from build123d import *

# Parameters (mm, degrees)
BOSS_EXTRUDE1_DEPTH = 1.5875
CUT_EXTRUDE1_DEPTH  = 3.175
FILLET1_R           = 8.89


with BuildPart() as part:
    # Sketch1 → Boss-Extrude1 (new, symmetric)
    with BuildSketch(Plane.XY):
        with BuildLine():
            Line((-120.187952283, -34.272453), (-93.24718392, -61.213221363))
            Line((-93.24718392, -61.213221363), (-94.292689271, -70.797689271))
            ThreePointArc((-94.292689271, -70.797689271), (-77.124658044, -85.289234251), (-57.767453, -96.692952283))
            ThreePointArc((-57.767453, -96.692952283), (94.292689271, 117.787689271), (-120.187952283, -34.272453))
        make_face()
    extrude(amount=BOSS_EXTRUDE1_DEPTH, both=True)

    # Sketch2 → Cut-Extrude1 (cut)
    with BuildSketch(Plane.XY.offset(1.5875)):
        with BuildLine():
            Line((-77.304798152, -55.60299244), (-78.320318415, -64.912577861))
            ThreePointArc((-78.320318415, -64.912577861), (94.997930523, 93.675946819), (-107.51910025, -25.388690342))
            Line((-107.51910025, -25.388690342), (-77.304798152, -55.60299244))
        make_face()
    extrude(amount=-CUT_EXTRUDE1_DEPTH, mode=Mode.SUBTRACT)

    # Fillet1
    fillet1_edges = [part.edges().sort_by_distance(p)[0] for p in [
        (-77.304798152, -55.60299244, 0),
        (-107.51910025, -25.388690342, 0),
        (-78.320318415, -64.912577861, 0),
        (-93.24718392, -61.213221363, -0.79375),
        (-120.187952283, -34.272453, -0.79375),
        (-94.292689271, -70.797689271, -0.79375),
    ]]
    fillet(fillet1_edges, radius=FILLET1_R)


solid = part.part
Build history of the part. All positions in model axes, mm. Coordinates: 2 decimals unless noted, no trailing zeros. Order: outer loops, then holes, each group sorted by start corner. A loop starts at its lowest first (then second) coordinate and runs counter-clockwise, first axis right, second up. Notation, with made-up numbers: (65, 36) - (100, 36) arc R14 cw to (100, 58) - close; hole circle Ø7 at (25.5, -22.75). An arc over 180 degrees is marked (long way). Write item = value, one per line. Start each with the question number.
1) Wall check: line 1 along Y through (x, z) = (0, -0.05) (3 decimals); line 2 along X through (y, z) = (105, 0.75); line 3 along Y through (x, z) = (83.5, -1.4). Give the ranges that are in metal, low to high. Write a range as from..to.
2) Saw through at A-A on x = -34.5. Write the cut outline in (y, z).
3) Two-plate mould, pull along Y, no slides. Class faces 1 (the face through (-93.52, -39.39, 0.02)), 2 (the face through (-80, -55, -1.588)), 3 (the face through (-107.84, -46.62, 0.02)): pulls with the +Y half, pulls with the -Y half, needs draft (parallel to the pull), parting line crosses it, or undercut.
4) Flat gauge pin, fed straight in: pin 1 Ø1.5 at (y, z) = (-5.5, 0.5) entering from +X. Where does the tip first touch, or does it go through?
5) Saw through at B-B on y = 36. Write the cut outline in (x, z), then the cut area to 3 significant figures.
From the geometry:
q1.line_1 = -109.855..-94.615, 141.605..156.845
q1.line_2 = -105.54..-85.48, 85.48..105.54
q1.line_3 = -80.48..-60.04, 107.03..127.47
q2.outline = (-105.31, -1.59) - (-89.46, -1.59) - (-89.46, 1.59) - (-105.31, 1.59) - close; (136.45, -1.59) - (152.3, -1.59) - (152.3, 1.59) - (136.45, 1.59) - close
q3.face_1 = undercut
q3.face_2 = needs draft
q3.face_3 = pulls with the -Y half
q4.pin_1 = 130.32
q5.outline = (-132.76, -1.59) - (-117.45, -1.59) - (-117.45, 1.59) - (-132.76, 1.59) - close; (117.45, -1.59) - (132.76, -1.59) - (132.76, 1.59) - (117.45, 1.59) - close
q5.area = 97.3 mm^2
